Autodesk Fusion 360 part; units mm, degrees
sketch "Sketch1" plane through (0, 0, 0) normal (1, 0, 0) x (0, 1, 0)
  line L0 (0, 0) -> (80, 0)
  line L1 (80, 0) -> (80, -50)
  line L2 (80, -50) -> (0, -50)
  line L3 (0, -50) -> (0, 0)
  arc A0 (0, -50) -> (80, -50) centre (40, -50) ccw
  circle A1 centre (40, -50) radius 16
sketch "Sketch2" plane through (0, 0, 0) normal (1, 0, 0) x (0, 1, 0)
extrude "Extrude1" add sketch "Sketch1" along normal blind 120 contours L0 L1 L2 L3 A1 | L2 A0 A1
sketch "Sketch3" plane through (0, 0, 0) normal (1, 0, 0) x (0, 1, 0)
sketch "Sketch4" plane through (0, 0, 0) normal (0, -1, 0) x (1, 0, 0)
  line L0 (0, 0) -> (0, -50)
  line L1 (0, -50) -> (120, -50)
  line L2 (120, -50) -> (120, 0)
  line L3 (120, 0) -> (0, 0)
  line L4 (0, 0) -> (20, 0)
  line L5 (0, 0) -> (0, -15)
  line L6 (20, -14.9206) -> (100, -14.9206)
  line L7 (100, -14.9206) -> (100, -90)
  line L8 (100, -90) -> (20, -90)
  line L9 (20, -90) -> (20, -14.9206)
  dimension "d3" = 20
  dimension "d4" = 15
extrude "Extrude2" cut sketch "Sketch4" against normal blind 90 contours L1 L6 L7 L9 | L1 L7 L8 L9
sketch "Sketch5" plane through (0, 0, 0) normal (0, 0, 1) x (-1, 0, 0)
  line L0 (0, -80) -> (0, 0)
  line L1 (0, 0) -> (-120, 0)
  line L2 (-120, 0) -> (-120, -80)
  line L3 (-120, -80) -> (0, -80)
sketch "Sketch6" plane through (0, 0, 0) normal (0, 0, 1) x (-1, 0, 0)
  circle A0 centre (-60, -40) radius 40
  circle A1 centre (-60, -40) radius 30
  circle A2 centre (-60, -40) radius 15
  dimension "d7" = 60
  dimension "d8" = 30
extrude "Extrude4" cut sketch "Sketch6" against normal blind 25 contours A2
extrude "Extrude5" add sketch "Sketch6" along normal blind 5 contours A1
extrude "Extrude6" add sketch "Sketch6" along normal blind 20 contours A0
extrude "Extrude3" [suppressed]
sketch "Sketch7" plane through (0, 0, 0) normal (0, 0, 1) x (-1, 0, 0)
Model file for the job. Use its own axes, mm. A direction names the side the tool comes from. Coordinates: 2 decimals unless noted, no trailing zeros. Order: outer loops, then holes, each group sorted by start corner. A loop starts at its lowest first (then second) coordinate and runs counter-clockwise, first axis right, second up. Notation, with made-up numbers: (2, 40) -> (27, 40) arc R19 cw to (27, 66) -> close; hole circle Ø10 at (62.25, -28.75). An arc over 180 degrees is marked (long way). Answer as a JSON object with one key per item and string values. Group by question number.
1) Cut at D-D, the plane z = -38.5. Write the cut outline in (x, y).
2) Cut at A-A, the plane z = -19. Write the cut outline in (x, y), then the cut area to 3 significant figures.
3) Flat gauge pins, fed straight in: pin 1 (18 mm diameter, centred on x = 41, y = 45.5, fed in from +Z); pin 2 (3 mm diameter, centred on x = 104, y = 50.5, fed in from +Z); pin 3 (8 mm diameter, centred on x = 17, y = 42.5, fed in from -Z). Where does each tip first touch, or does it go through?
4) Cut at C-C, the plane x = 109.5. Write the cut outline in (y, z).
5) Drill centre lines: L1, parallel to Y at x = 60, z = 13.5; L2, parallel to Y at x = 60, z = 0.75; L3, parallel to X at y = 61.5, z = -42. Where is each one in solid material? Low to high.
6) Cut at B-B, the plane y = 40. Write the cut outline in (x, z), then the cut area to 3 significant figures.
7) Which spindle directions (+Z, -Z, +X, -X, +Y, -Y) get a long thin tool onto all of the face, cutting with end or side? Do faces 1 (the face through (100, 48, -35)), 2 (the face through (103, 39, 0)), 3 (the face through (109.86, 28.207, -60.814)), 4 (the face through (74, 46, 5)), 5 (the face through (109.86, 40.88, -89.99)). Say none if no direction does.
8) Pull direction Z, two halves, no side cores. Call faces 6 (the face through (59, 80, -14)), 7 (the face through (16, 39, 0)), 8 (the face through (9.86, 28.207, -60.814)): +Z half, -Z half, draft (parallel to the pull), parting line (faces both ways), or undercut.
Check values:
{
 "1": {"outline": "(0, 0) -> (20, 0) -> (20, 28.88) -> (0, 28.88) -> close; (0, 51.12) -> (20, 51.12) -> (20, 80) -> (0, 80) -> close; (100, 0) -> (120, 0) -> (120, 28.88) -> (100, 28.88) -> close; (100, 51.12) -> (120, 51.12) -> (120, 80) -> (100, 80) -> close"},
 "2": {"outline": "(0, 0) -> (20, 0) -> (20, 80) -> (0, 80) -> close; (100, 0) -> (120, 0) -> (120, 80) -> (100, 80) -> close", "area": "3,200 mm²"},
 "3": {"pin 1": "stops at z = 5", "pin 2": "stops at z = 0", "pin 3": "stops at z = -90"},
 "4": {"outline": "(0, -50) arc R40 ccw to (80, -50) -> (80, 0) -> (0, 0) -> close; hole circle Ø32 at (40, -50)"},
 "5": {"L1": "y = 0 to 10, 70 to 80", "L2": "y = 0 to 25, 55 to 80", "L3": "x = 0 to 20, 100 to 120"},
 "6": {"outline": "(0, -90) -> (20, -90) -> (20, -66) -> (0, -66) -> close; (0, -34) -> (20, -34) -> (20, -14.92) -> (45, -14.92) -> (45, 5) -> (30, 5) -> (30, 20) -> (20, 20) -> (20, 0) -> (0, 0) -> close; (75, -14.92) -> (100, -14.92) -> (100, -34) -> (120, -34) -> (120, 0) -> (100, 0) -> (100, 20) -> (90, 20) -> (90, 5) -> (75, 5) -> close; (100, -90) -> (120, -90) -> (120, -66) -> (100, -66) -> close", "area": "3,620 mm²"},
 "7": {"face 1": "-Z, +Y, -Y", "face 2": "+Z, +X", "face 3": "+X, -X", "face 4": "+Z", "face 5": "-Z, +X, -X"},
 "8": {"face 6": "draft", "face 7": "+Z half", "face 8": "undercut"}
}
